from build123d import *

# Parameters (mm, degrees)
SKETCH1_W                                      = 10
SKETCH1_H                                      = 13
EXTRUDE1_DEPTH                                 = 2.175
SKETCH3_W                                      = 7.9
SKETCH3_H                                      = 7.9
EXTRUDE3_DEPTH                                 = 1
CBORE_FOR_0_SOCKET_HEAD_CAP_SCREW1_D           = 1.778
CBORE_FOR_0_SOCKET_HEAD_CAP_SCREW1_CBORE_D     = 3.175
CBORE_FOR_0_SOCKET_HEAD_CAP_SCREW1_CBORE_DEPTH = 1.524
F_3_32_0_09375_DIAMETER_HOLE1_D                = 2.38125
F_3_32_0_09375_DIAMETER_HOLE1_DEPTH            = 10
F_3_32_0_09375_DIAMETER_HOLE1_TIP              = 0.715399675
FILLET3_R                                      = 1


with BuildPart() as part:
    # Sketch1 → Extrude1 (new body)
    with BuildSketch(Plane(origin=(0, 0, 0), x_dir=(1, 0, 0), z_dir=(0, 1, 0))):
        Rectangle(SKETCH1_W, SKETCH1_H)
    extrude(amount=EXTRUDE1_DEPTH)

    # Sketch3 → Extrude3 (add)
    with BuildSketch(Plane(origin=(0, 2.175, 0), x_dir=(1, 0, 0), z_dir=(0, 1, 0))):
        with Locations((0, -1.5)):
            Rectangle(SKETCH3_W, SKETCH3_H)
    extrude(amount=EXTRUDE3_DEPTH)

    # CBORE for #0 Socket Head Cap Screw1 (through all)
    with Locations(Plane(origin=(0, 0, -4.5), x_dir=(0, 0, -1), z_dir=(0, -1, 0))):
        with Locations((0, 0)):
            CounterBoreHole(CBORE_FOR_0_SOCKET_HEAD_CAP_SCREW1_D / 2, CBORE_FOR_0_SOCKET_HEAD_CAP_SCREW1_CBORE_D / 2, CBORE_FOR_0_SOCKET_HEAD_CAP_SCREW1_CBORE_DEPTH)

    # 3/32 (0.09375) Diameter Hole1
    with Locations(Plane(origin=(-3, 0, -4.5), x_dir=(0, 0, -1), z_dir=(0, -1, 0))):
        with Locations((0, 0), (0, 6)):
            Hole(F_3_32_0_09375_DIAMETER_HOLE1_D / 2, depth=F_3_32_0_09375_DIAMETER_HOLE1_DEPTH)
            with Locations((0, 0, -(F_3_32_0_09375_DIAMETER_HOLE1_DEPTH + F_3_32_0_09375_DIAMETER_HOLE1_TIP / 2))):  # 118° drill point
                Cone(0, F_3_32_0_09375_DIAMETER_HOLE1_D / 2, F_3_32_0_09375_DIAMETER_HOLE1_TIP, mode=Mode.SUBTRACT)

    # Fillet3
    # the kernel refuses this fillet: 1 mm, written as the material it takes off along each edge
    with BuildSketch(Plane(origin=(-4, 1, -5.5), x_dir=(0, -1, 0), z_dir=(-1, 0, 0))) as fillet3_piece_1_section:
        Polygon((0, 0), (FILLET3_R, 0), (FILLET3_R, -FILLET3_R), (0, -FILLET3_R), align=None)
    fillet3_piece_1 = extrude(amount=FILLET3_R, mode=Mode.PRIVATE)
    fillet3_piece_1 = fillet3_piece_1 - Plane(origin=(-4, 1, -5.5), x_dir=(0, 0.7071067811865475, 0.7071067811865475), z_dir=(-1, 0, 0)) * Sphere(FILLET3_R, mode=Mode.PRIVATE)
    add(fillet3_piece_1, mode=Mode.SUBTRACT)
    with BuildSketch(Plane(origin=(4, 1, -5.5), x_dir=(0, -1, 0), z_dir=(1, 0, 0))) as fillet3_piece_2_section:
        Polygon((0, 0), (FILLET3_R, 0), (FILLET3_R, FILLET3_R), (0, FILLET3_R), align=None)
    fillet3_piece_2 = extrude(amount=FILLET3_R, mode=Mode.PRIVATE)
    fillet3_piece_2 = fillet3_piece_2 - Plane(origin=(4, 1, -5.5), x_dir=(0, 0.7071067811865475, 0.7071067811865475), z_dir=(1, 0, 0)) * Sphere(FILLET3_R, mode=Mode.PRIVATE)
    add(fillet3_piece_2, mode=Mode.SUBTRACT)
    with BuildSketch(Plane(origin=(4, 1, 5.5), x_dir=(1, 0, 0), z_dir=(0, 0, 1))) as fillet3_piece_3_section:
        Polygon((0, 0), (FILLET3_R, 0), (FILLET3_R, -FILLET3_R), (0, -FILLET3_R), align=None)
    fillet3_piece_3 = extrude(amount=FILLET3_R, mode=Mode.PRIVATE)
    fillet3_piece_3 = fillet3_piece_3 - Plane(origin=(4, 1, 5.5), x_dir=(-0.7071067811865475, 0.7071067811865475, 0), z_dir=(0, 0, 1)) * Sphere(FILLET3_R, mode=Mode.PRIVATE)
    add(fillet3_piece_3, mode=Mode.SUBTRACT)
    with BuildSketch(Plane(origin=(-4, 1, 5.5), x_dir=(-1, 0, 0), z_dir=(0, 0, 1))) as fillet3_piece_4_section:
        Polygon((0, 0), (FILLET3_R, 0), (FILLET3_R, FILLET3_R), (0, FILLET3_R), align=None)
    fillet3_piece_4 = extrude(amount=FILLET3_R, mode=Mode.PRIVATE)
    fillet3_piece_4 = fillet3_piece_4 - Plane(origin=(-4, 1, 5.5), x_dir=(0.7071067811865475, 0.7071067811865475, 0), z_dir=(0, 0, 1)) * Sphere(FILLET3_R, mode=Mode.PRIVATE)
    add(fillet3_piece_4, mode=Mode.SUBTRACT)
    with BuildSketch(Plane(origin=(-3.95, 2.175, -2.45), x_dir=(0, 0, 1), z_dir=(0, 1, 0)), Plane(origin=(3.95, 2.175, -2.45), x_dir=(-1, 0, 0), z_dir=(0, 1, 0))) as fillet3_piece_5:
        with BuildLine():
            CenterArc((FILLET3_R, FILLET3_R), FILLET3_R, 180, 90)
            Line((0, FILLET3_R), (0, 0))
            Line((0, 0), (FILLET3_R, 0))
        make_face()
    extrude(amount=3.5, mode=Mode.SUBTRACT)
    with BuildSketch(Plane(origin=(-3.95, 2.175, 5.45), x_dir=(0, 0, -1), z_dir=(0, 1, 0)), Plane(origin=(3.95, 2.175, 5.45), x_dir=(-1, 0, 0), z_dir=(0, 1, 0))) as fillet3_piece_6:
        with BuildLine():
            CenterArc((FILLET3_R, -FILLET3_R), FILLET3_R, 90, 90)
            Line((0, -FILLET3_R), (0, 0))
            Line((0, 0), (FILLET3_R, 0))
        make_face()
    extrude(amount=3.5, mode=Mode.SUBTRACT)
    with BuildSketch(Plane(origin=(-4, 0, -6.5), x_dir=(0, 0, 1), z_dir=(1, 0, 0))) as fillet3_piece_7:
        with BuildLine():
            CenterArc((FILLET3_R, -FILLET3_R), FILLET3_R, 90, 90)
            Line((0, -FILLET3_R), (0, 0))
            Line((0, 0), (FILLET3_R, 0))
        make_face()
    extrude(amount=8, mode=Mode.SUBTRACT)
    with BuildSketch(Plane(origin=(5, 0, -5.5), x_dir=(0, 1, 0), z_dir=(0, 0, 1)), Plane(origin=(-5, 0, 5.5), x_dir=(0, 1, 0), z_dir=(0, 0, -1))) as fillet3_piece_8:
        with BuildLine():
            CenterArc((FILLET3_R, FILLET3_R), FILLET3_R, 180, 90)
            Line((0, FILLET3_R), (0, 0))
            Line((0, 0), (FILLET3_R, 0))
        make_face()
    extrude(amount=11, mode=Mode.SUBTRACT)
    with BuildSketch(Plane(origin=(4, 0, 6.5), x_dir=(0, 1, 0), z_dir=(-1, 0, 0))) as fillet3_piece_9:
        with BuildLine():
            CenterArc((FILLET3_R, FILLET3_R), FILLET3_R, 180, 90)
            Line((0, FILLET3_R), (0, 0))
            Line((0, 0), (FILLET3_R, 0))
        make_face()
    extrude(amount=8, mode=Mode.SUBTRACT)
    with BuildSketch(Plane(origin=(-5, 1, -6.5), x_dir=(0, 0, 1), z_dir=(0, 1, 0)), Plane(origin=(-5, 1, 6.5), x_dir=(1, 0, 0), z_dir=(0, 1, 0))) as fillet3_piece_10:
        with BuildLine():
            CenterArc((FILLET3_R, FILLET3_R), FILLET3_R, 180, 90)
            Line((0, FILLET3_R), (0, 0))
            Line((0, 0), (FILLET3_R, 0))
        make_face()
    extrude(amount=3.675, mode=Mode.SUBTRACT)
    with BuildSketch(Plane(origin=(5, 1, -6.5), x_dir=(0, 0, 1), z_dir=(0, 1, 0)), Plane(origin=(5, 1, 6.5), x_dir=(-1, 0, 0), z_dir=(0, 1, 0))) as fillet3_piece_11:
        with BuildLine():
            CenterArc((FILLET3_R, -FILLET3_R), FILLET3_R, 90, 90)
            Line((0, -FILLET3_R), (0, 0))
            Line((0, 0), (FILLET3_R, 0))
        make_face()
    extrude(amount=3.675, mode=Mode.SUBTRACT)


solid = part.part
Verification items for the finished model (mm, model axes). A direction names the side the tool comes from. Give positions to 0.01 mm unless a question says otherwise; leave off trailing zeros. Loops run counter-clockwise (first coordinate to the right, second up) from the corner with the lowest first, then second, coordinate; pieces in that order, holes last.
1. Cross-section at C-C on z = 4. Record the cut outline in (x, y) (3 decimals).
Derived:
outline: (-5, 1) arc R1 ccw to (-4, 0) - (4, 0) arc R1 ccw to (5, 1) - (5, 2.175) - (3.95, 2.175) - (3.95, 3.175) - (-3.95, 3.175) - (-3.95, 2.175) - (-5, 2.175) - close
2. Cross-section at B-B on z = -4.5. Count the separate pieces of the cut face and the enclosed holes in it, and give its area (3 significant figures).
Derived:
separate pieces: 4
enclosed holes: 0
area: 4.97 mm2
3. Release check for a two-part mould opening along Z. For faces 6 (the flat face through (3.95, 3, 2)), 7 (the cylindrical face through (-4.715, 1.579, 6.199)), 8 (the cylindrical face through (2.276, 1.103, -5.445)), 9 (the cylindrical face through (-3.649, 2.668, -2.165)) record: +Z half, -Z half, draft (parallel to the pull), parting line (faces both ways), or undercut.
Derived:
face 6: draft
face 7: +Z half
face 8: undercut
face 9: -Z half
4. Material ranges on probe 1 along X at (y, z) = (1.65, -4.5); probe 2 along X at (y, z) = (1.15, -4.5); probe 3 along Z at (x, y) = (-3, 1.65), recorded low to high.
Derived:
probe 1: x = -5 to -4.19, -1.81 to -0.89, 0.89 to 1.81, 4.19 to 5
probe 2: x = -5 to -4.19, -1.81 to -1.59, 1.59 to 1.81, 4.19 to 5
probe 3: z = -6.5 to -5.69, -3.31 to 6.5
5. Tool access check on faces 1 (the flat face through (-3.95, 3, 2)), 2 (the flat face through (-1, 1.524, -5)), 3 (the cylindrical face through (3.665, 2.668, -2.149)), 4 (the cylindrical face through (3.649, 2.668, 5.165)), 5 (the flat face through (0, 3, -2.45)). Record the directions out of +Z, -Z, +X, -X, +Y, -Y that give a thin tool (end or side, any length) a straight path to the whole face; none if there is none.
Derived:
face 1: +Z, -Z, -X, +Y
face 2: -Y
face 3: -Z, +X, +Y
face 4: +Z, +X, +Y
face 5: -Z, +X, -X, +Y
6. Go/stop test with flat-tipped pins: P1, Ø2, axis at x = 3, z = -4.5, coming from the -Y side; P2, Ø0.5, axis at y = 3, z = 1, coming from the +X side; P3, Ø1.6, axis at x = 0, z = -5, coming from the -Y side; P4, Ø0.8, axis at x = -0.5, y = 3, coming from the +Z side. Record where each tip stops, or that it passes through.
Derived:
P1: passes through
P2: stops at x = 3.95
P3: stops at y = 1.52
P4: stops at z = 5.45
7. Cross-section at A-A on x = 2.75. Record the cut outline in (y, z) (3 decimals), and give its area (3 significant figures).
Derived:
outline: (0, -3.336) - (2.175, -3.336) - (2.175, -2.45) - (3.175, -2.45) - (3.175, 5.45) - (2.175, 5.45) - (2.175, 6.5) - (1, 6.5) arc R1 ccw to (0, 5.5) - close; (0.014, -5.664) arc R1 ccw to (1, -6.5) - (2.175, -6.5) - (2.175, -5.664) - close
area: 30.7 mm2
8. Cross-section at D-D on y = 0.8. Record the cut outline in (x, z) (1 decimal), and give its area (3 significant figures).
Derived:
outline: (-5, -5.5) arc R1 ccw to (-4, -6.5) - (4, -6.5) arc R1 ccw to (5, -5.5) - (5, 5.5) arc R1 ccw to (4, 6.5) - (-4, 6.5) arc R1 ccw to (-5, 5.5) - close; hole circle Ø2.4 at (-3, -4.5); hole circle Ø3.2 at (0, -4.5); hole circle Ø2.4 at (3, -4.5)
area: 111 mm2
